The listing builds one solid part. Answer for the finished solid, in the listing's coordinates (mm). A direction names the side the tool comes from. Give positions to 0.01 mm unless a question says otherwise; leave off trailing zeros. Order: outer loops, then holes, each group sorted by start corner. A loop starts at its lowest first (then second) coordinate and runs counter-clockwise, first axis right, second up.
```python
from build123d import *

# Parameters (mm, degrees)
F2_SIZE  = 0.4
F3_R     = 0.4
F4_SIZE2 = 0.3349364905
F4_SIZE  = 1.25


with BuildPart() as f1:
    # F0 (on Top) → F1 (revolve)
    with BuildSketch(Plane.XY):
        Polygon((-22.8699422013, 6.35), (-22.8699422013, 2.8), (23.7300577987, 2.8), (23.7300577987, 7.35), (-1.1699422013, 7.35), (-1.1699422013, 13.2), (-1.5699422013, 13.2), (-1.5699422013, 22.2), (-7.2699422013, 22.2), (-7.2699422013, 9.25), (-7.4699422013, 9.25), (-7.4699422013, 6.35), align=None)
    revolve(axis=Axis((0.339884735, 0, 0), (1, 0, 0)))

    # F2
    f2_edges = [f1.edges().sort_by_distance(p)[0] for p in [
        (23.730058, -7.35, 0),
        (-22.869942, -6.35, 0),
        (-22.869942, -2.8, 0),
        (23.730058, -2.8, 0),
    ]]
    chamfer(f2_edges, length=F2_SIZE)

    # F3
    f3_edges = [f1.edges().sort_by_distance(p)[0] for p in [
        (-7.469942, -6.35, 0),
        (-1.169942, -7.35, 0),
    ]]
    fillet(f3_edges, radius=F3_R)

    # F4
    f4_edges = [f1.edges().sort_by_distance(p)[0] for p in [
        (-1.569942, -22.2, 0),
        (-7.269942, -22.2, 0),
    ]]
    f4_side = f1.faces().sort_by_distance((-4.419942, -22.2, 0))[0]
    chamfer(f4_edges, length=F4_SIZE, length2=F4_SIZE2, reference=f4_side)


solid = f1.part
```
1) Find section B-B (x = -19). Write down the section's boundary in (y, z), then the cut area to 3 significant figures.
Geometry says:
outline: circle Ø12.7 at (0, 0); hole circle Ø5.6 at (0, 0)
area: 102 mm2
2) For a pull along Z with two mould halves and no side action, classify faces 1 (the cylindrical face through (-1.37, -9.73, 8.92)), 2 (the flat face through (-22.87, 3, -3)), 3 (the cylindrical face through (0.8, -2.8, 0.1)) as +Z half, -Z half, draft (parallel to the pull), parting line (faces both ways), or undercut.
Geometry says:
face 1: parting line
face 2: draft
face 3: undercut
3) A tool of negligible diameter and unlimited length cuts with its end or side. For faces 4 (the flat face through (-1.57, 0, -14)), 5 (the cylindrical face through (-4.44, 11.93, 18.72)), 6 (the flat face through (-7.47, 1, -7)), from which of +Z, -Z, +X, -X, +Y, -Y can it reach the whole face along a straight path? Write none if from no direction.
Geometry says:
face 4: +X
face 5: +X, -X
face 6: -X
4) Straight lines are drawn through the part: probe 1 along Z at (x, y) = (13, 0); probe 2 along Z at (x, y) = (-10.5, 0); probe 3 along X at (y, z) = (-7, -12.5). For each, find the intervals that lie inside material, in ascending order.
Geometry says:
probe 1: z = -7.35 to -2.8, 2.8 to 7.35
probe 2: z = -6.35 to -2.8, 2.8 to 6.35
probe 3: x = -7.27 to -1.57
5) Given P1, Ø5, axis at y = -7.5, z = -2, coming from the +X side; P2, Ø6, axis at x = -2.5, z = 7.5, coming from the -Y side; P3, Ø4, axis at x = -16.5, z = 0, coming from the -Y side; P4, Ø3.5, axis at y = 0, z = 0, coming from the -X side, each flat-ended and moving along its own axis, determine where each tip first touches the part or whether it passes through.
Geometry says:
P1: stops at x = 23.73
P2: stops at y = -21.74
P3: stops at y = -6.35
P4: passes through
6) Find section A-A (x = 1). Write down the section's boundary in (y, z), then the cut area to 3 significant figures.
Geometry says:
outline: circle Ø14.7 at (0, 0); hole circle Ø5.6 at (0, 0)
area: 145 mm2
